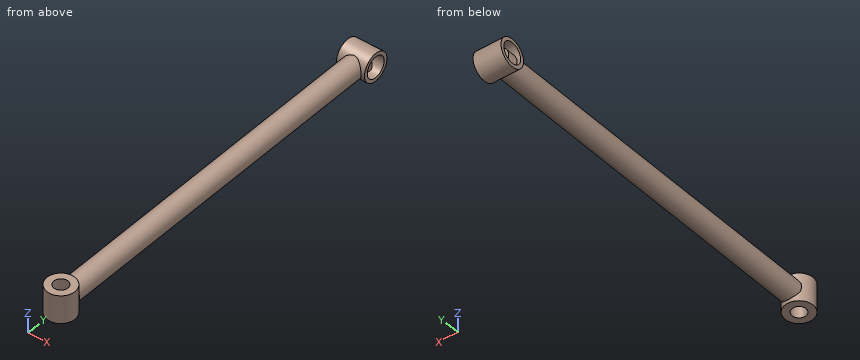
```python
from build123d import *

# Parameters (mm, degrees)
F1_R     = 12.7
F1_R_2   = 9.525
F2_DEPTH = 12.7
F0_R     = 9.525
F3_DEPTH = 330.2
F4_R     = 12.7
F4_R_2   = 6.35
F5_DEPTH = 12.7


with BuildPart() as f2:
    # F1 (on Right) → F2 (new body, symmetric)
    with BuildSketch(Plane.YZ):
        Circle(F1_R)
        Circle(F1_R_2, mode=Mode.SUBTRACT)
    extrude(amount=F2_DEPTH, both=True)

    # F0 (on Front) → F3 (join)
    with BuildSketch(Plane.XZ):
        Circle(F0_R)
    extrude(amount=F3_DEPTH)

    # F4 (on Top) → F5 (join, symmetric)
    with BuildSketch(Plane.XY):
        with Locations((0, -339.3217325211)):
            Circle(F4_R)
        with Locations((0, -339.3217325211)):
            Circle(F4_R_2, mode=Mode.SUBTRACT)
    extrude(amount=F5_DEPTH, both=True)


solid = f2.part
```
Source: CAD feature listing. Evaluate the final solid. Frame: model axes, mm. Round coordinates to 2 decimals unless told otherwise and drop trailing zeros. Loops run counter-clockwise (first coordinate to the right, second up) from the corner with the lowest first, then second, coordinate; pieces in that order, holes last. Notation, with made-up numbers: M 11,13 L 26,13 A24 ccw 26,52 Z; hole C -11.75,60.5 d11. An arc over 180 degrees is marked long. Use a Markdown table: item, result. Add a question column.
1. Section query A-A on z = 0. Return the cut outline in (x, y) (3 decimals).
2. Line query: line 1 (Y direction, x = 0, z = -0.5); line 2 (Y direction, x = -0.75, z = 0) (3 decimals); line 3 (Z direction, x = 3.5, y = -204.5). Output: solid intervals per line, ascending.
3. Contact query for flat-ended pins moving along their axis: P1, Ø3, axis at x = 0, y = -256, coming from the +Z side (3 decimals); P2, Ø10, axis at y = -237.5, z = -3.5, coming from the +X side (3 decimals); P3, Ø0.8, axis at x = 9, z = 1.5, coming from the -Y side; P4, Ø9.5, axis at x = 2.5, z = -4.5, coming from the +Y side. Output: stop coordinate, or through.
4. Section query B-B on y = -322. Return the cut outline in (x, z) (3 decimals).
Reported:
| question | item | result |
|---|---|---|
| 1 | outline | M -12.7,-12.7 L -9.525,-12.7 L -9.525,-330.2 L -8.837,-330.2 A12.7 ccw long 8.837,-330.2 L 9.525,-330.2 L 9.525,-12.7 L 12.7,-12.7 L 12.7,-9.525 L 9.525,-9.525 L 9.525,0 L -9.525,0 L -9.525,-9.525 L -12.7,-9.525 Z; M -12.7,9.525 L 12.7,9.525 L 12.7,12.7 L -12.7,12.7 Z; hole C 0,-339.322 d12.7 |
| 2 | line 1 | y = -352.02 to -345.67, -332.97 to 0, 9.51 to 12.69 |
| 2 | line 2 | y = -352 to -345.627, -333.016 to 0, 9.525 to 12.7 |
| 2 | line 3 | z = -8.86 to 8.86 |
| 3 | P1 | stops at z = 9.525 |
| 3 | P2 | stops at x = 9.525 |
| 3 | P3 | stops at y = -348.67 |
| 3 | P4 | stops at y = 12.7 |
| 4 | outline | C 0,0 d19.05 |
